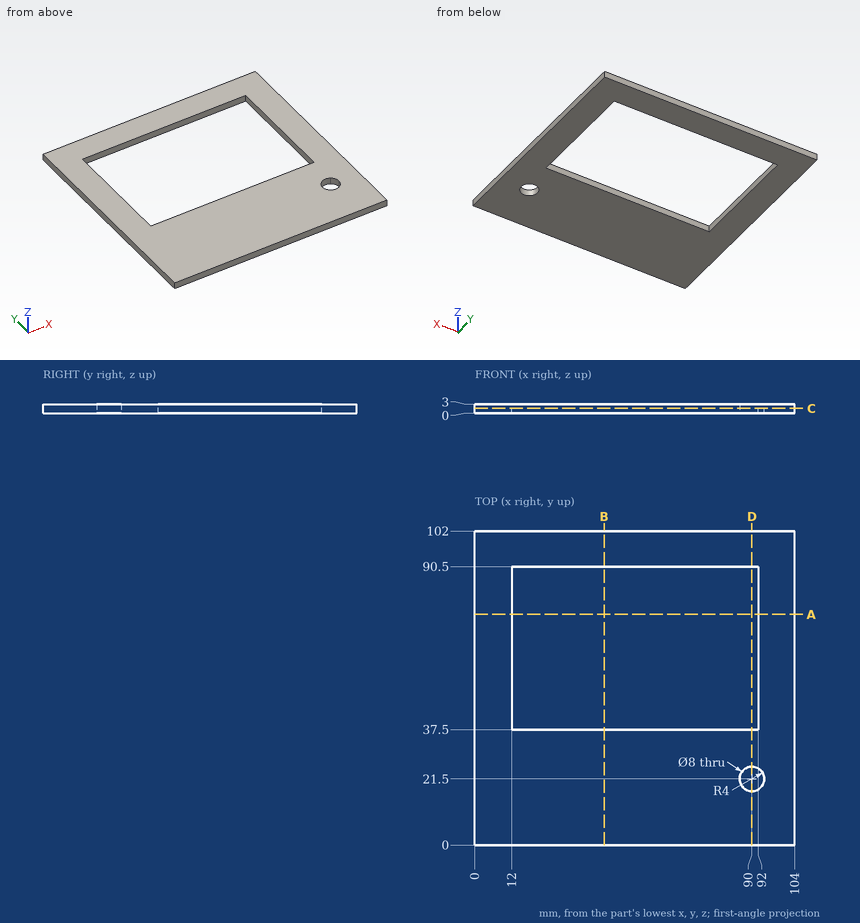
Source: three-view drawing plus pictorial views. Frame: mm from the lowest corner of the part. Give positions to 0.01 mm unless a question says otherwise; leave off trailing zeros. Order: outer loops, then holes, each group sorted by start corner. A loop starts at its lowest first (then second) coordinate and runs counter-clockwise, first axis right, second up. Notation, with made-up numbers: (29, 15) -> (63, 15) arc R10 ccw to (63, 32) -> close; hole circle Ø5 at (2.5, 82.25). An arc over 180 degrees is marked (long way). Use a Markdown table: item, result.
Q1. Section A-A (y = 75). Return the cut outline in (x, z), and give its area (3 significant figures).
A:
| item | result |
|---|---|
| outline | (0, 0) -> (12, 0) -> (12, 3) -> (0, 3) -> close; (92, 0) -> (104, 0) -> (104, 3) -> (92, 3) -> close |
| area | 72.0 mm^2 |
Q2. Section C-C (z = 1.55). Return the cut outline in (x, y), and give its area (3 significant figures).
A:
| item | result |
|---|---|
| outline | (0, 0) -> (104, 0) -> (104, 102) -> (0, 102) -> close; hole (12, 37.5) -> (92, 37.5) -> (92, 90.5) -> (12, 90.5) -> close; hole (92, 24.96) arc R4 ccw (long way) to (94, 21.5) arc R4 ccw to start |
| area | 6,320 mm^2 |
Q3. Section B-B (x = 42). Return the cut outline in (y, z), and give its area (3 significant figures).
A:
| item | result |
|---|---|
| outline | (0, 0) -> (37.5, 0) -> (37.5, 3) -> (0, 3) -> close; (90.5, 0) -> (102, 0) -> (102, 3) -> (90.5, 3) -> close |
| area | 147 mm^2 |
Q4. Material intervals for line 1 (Y direction, x = 90, z = 1.8); line 2 (Y direction, x = 74, z = 1.2); line 3 (X direction, y = 62, z = 0.5), sorted ascending. Write a range as [from, to].
A:
| item | result |
|---|---|
| line 1 | [0, 17.5], [25.5, 37.5], [90.5, 102] |
| line 2 | [0, 37.5], [90.5, 102] |
| line 3 | [0, 12], [92, 104] |
Q5. Section D-D (x = 90). Return the cut outline in (y, z), and give its area (3 significant figures).
A:
| item | result |
|---|---|
| outline | (0, 0) -> (17.5, 0) -> (17.5, 3) -> (0, 3) -> close; (25.5, 0) -> (37.5, 0) -> (37.5, 3) -> (25.5, 3) -> close; (90.5, 0) -> (102, 0) -> (102, 3) -> (90.5, 3) -> close |
| area | 123 mm^2 |
Q6. First-contact query: P1, Ø7, axis at x = 90, y = 21.5, coming from the +Z side. Flat tip, straight axial feed; report the tip coordinate or a pass-through.
A:
| item | result |
|---|---|
| P1 | through |
